Source: three-view drawing plus pictorial views. Frame: mm from the lowest corner of the part. Give positions to 0.01 mm unless a question says otherwise; leave off trailing zeros. Loops run counter-clockwise (first coordinate to the right, second up) from the corner with the lowest first, then second, coordinate; pieces in that order, holes last.
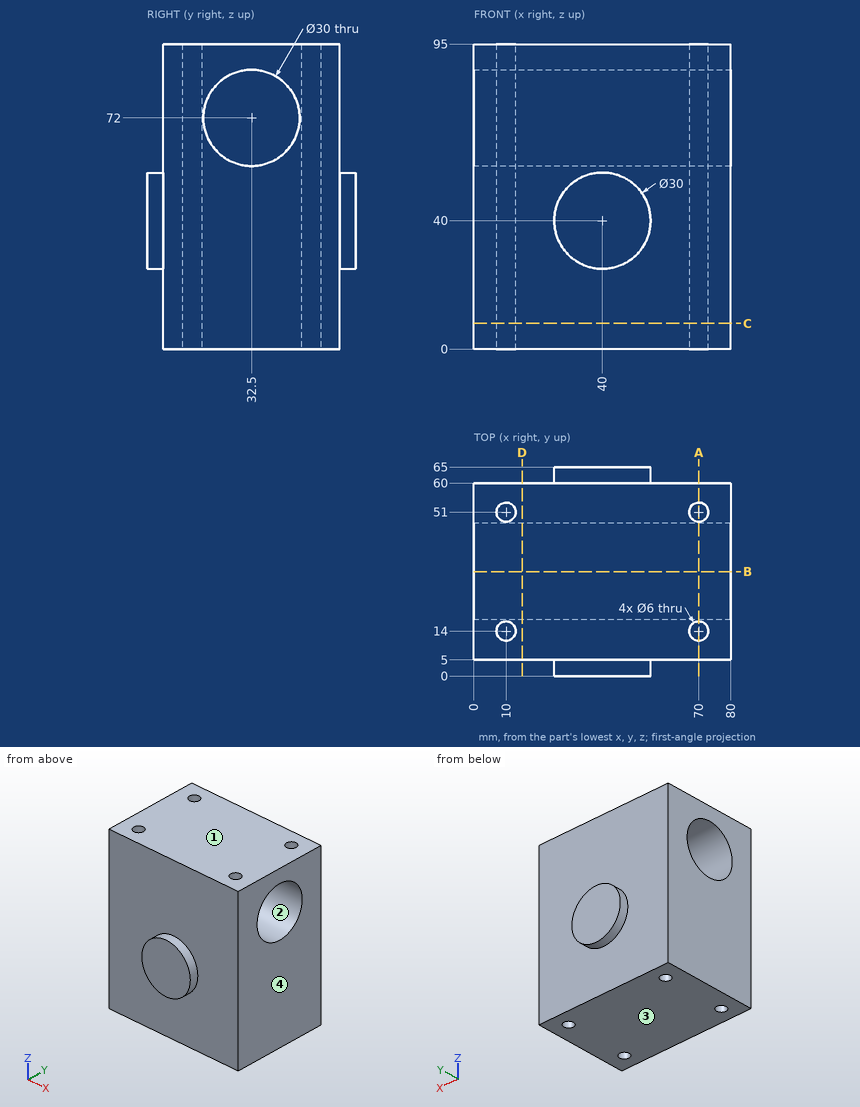
(1) Ray query, probe 1 along X at (y, z) = (14, 72); probe 2 along Y at (x, z) = (70, 16); probe 3 along Y at (x, z) = (12.5, 22.5). Return the intervals inside material, ascending.
Values follow:
probe 1: x = 0 to 7, 13 to 67, 73 to 80
probe 2: y = 5 to 11, 17 to 48, 54 to 60
probe 3: y = 5 to 12.34, 15.66 to 49.34, 52.66 to 60
(2) Cut plane C-C (z = 8). Return the cut outline in (x, y), and give its area (3 significant figures).
Values follow:
outline: (0, 5) - (80, 5) - (80, 60) - (0, 60) - close; hole circle Ø6 at (10, 14); hole circle Ø6 at (10, 51); hole circle Ø6 at (70, 14); hole circle Ø6 at (70, 51)
area: 4,290 mm2
(3) Mould query, pull axis Z, two halves, no side actions, for the marked faces 1, 2, 3 and 4. Classes: +Z half, -Z half, draft (parallel to the pull), parting line (faces both ways), or undercut.
Values follow:
face 1: +Z half
face 2: undercut
face 3: -Z half
face 4: draft
(4) Cut plane D-D (x = 15). Return the cut outline in (y, z).
Values follow:
outline: (5, 0) - (60, 0) - (60, 95) - (5, 95) - close; hole circle Ø30 at (32.5, 72)
(5) Cut plane A-A (x = 70). Return the cut outline in (y, z), and give its area (3 significant figures).
Values follow:
outline: (5, 0) - (11, 0) - (11, 95) - (5, 95) - close; (17, 0) - (48, 0) - (48, 95) - (17, 95) - close; (54, 0) - (60, 0) - (60, 95) - (54, 95) - close; hole circle Ø30 at (32.5, 72)
area: 3,380 mm2
(6) Pin query (flat end, axial travel): pin 1 Ø4 at (x, z) = (48.5, 76) entering from -Y. Return the tip coordinate at first contact, or that it passes through.
Values follow:
pin 1: stops at y = 5
(7) Cut plane B-B (y = 32.5). Return the cut outline in (x, z), and give its area (3 significant figures).
Values follow:
outline: (0, 0) - (80, 0) - (80, 57) - (0, 57) - close; (0, 87) - (80, 87) - (80, 95) - (0, 95) - close
area: 5,200 mm2
